```python
from build123d import *

# Parameters (mm, degrees)
SKETCH048_R     = 6.5
SKETCH048_R_2   = 3
PAD021_DEPTH    = 3.5
SKETCH049_R     = 5.5
SKETCH049_R_2   = 4
POCKET027_DEPTH = 0.5
SKETCH050_R     = 5.5
SKETCH050_R_2   = 4
POCKET028_DEPTH = 0.5


with BuildPart() as part:
    # Sketch048 → Pad021 (new body)
    with BuildSketch(Plane.XY):
        Circle(SKETCH048_R)
        Circle(SKETCH048_R_2, mode=Mode.SUBTRACT)
    extrude(amount=PAD021_DEPTH)

    # Sketch049 → Pocket027 (cut)
    with BuildSketch(Plane.XY.offset(3.5)):
        Circle(SKETCH049_R)
        Circle(SKETCH049_R_2, mode=Mode.SUBTRACT)
    extrude(amount=-POCKET027_DEPTH, mode=Mode.SUBTRACT)

    # Sketch050 → Pocket028 (cut)
    with BuildSketch(Plane.XY):
        Circle(SKETCH050_R)
        Circle(SKETCH050_R_2, mode=Mode.SUBTRACT)
    extrude(amount=POCKET028_DEPTH, mode=Mode.SUBTRACT)


solid = part.part
```
The listing builds one solid part. Answer for the finished solid, in the listing's coordinates (mm). A direction names the side the tool comes from. Give positions to 0.01 mm unless a question says otherwise; leave off trailing zeros. Order: outer loops, then holes, each group sorted by start corner. A loop starts at its lowest first (then second) coordinate and runs counter-clockwise, first axis right, second up.
1) Find section D-D on x = 4.25. Write down the section's boundary in (y, z), then the cut area to 3 significant figures.
Reported:
outline: (-4.92, 0) - (-3.49, 0) - (-3.49, 0.5) - (3.49, 0.5) - (3.49, 0) - (4.92, 0) - (4.92, 3.5) - (3.49, 3.5) - (3.49, 3) - (-3.49, 3) - (-3.49, 3.5) - (-4.92, 3.5) - close
area: 27.4 mm2
2) Consider line 1 along Y through (x, z) = (0, 0.35); line 2 along Z through (x, y) = (-5, 1.75); line 3 along X through (y, z) = (1.5, 3.1). Determine where each line is inside the solid, lowest interval first.
Reported:
line 1: y = -6.5 to -5.5, -4 to -3, 3 to 4, 5.5 to 6.5
line 2: z = 0.5 to 3
line 3: x = -6.32 to -5.29, -3.71 to -2.6, 2.6 to 3.71, 5.29 to 6.32
3) Given P1, Ø1, axis at y = -1, z = 1.5, coming from the +X side; P2, Ø1, axis at y = 1.5, z = 2.5, coming from the +X side; P3, Ø3.5, axis at x = 2, y = 2, coming from the -Z side, each flat-ended and moving along its own axis, determine where each tip first touches the part or whether it passes through.
Reported:
P1: stops at x = 6.48
P2: stops at x = 6.42
P3: stops at z = 0
4) Find section C-C on z = 3.2. Write down the section's boundary in (x, y).
Reported:
outline: circle Ø13 at (0, 0); circle Ø8 at (0, 0); hole circle Ø11 at (0, 0); hole circle Ø6 at (0, 0)
5) For faces 1 (the face through (-1.19, -5.37, 3.25)), 2 (the face through (-1.19, -5.37, 0.25)), 3 (the face through (1, 3, 0)), determine the directions among +Z, -Z, +X, -X, +Y, -Y from which every point of the face is accessible in a straight line to the end or side of a thin tool.
Reported:
face 1: +Z
face 2: -Z
face 3: -Z, +X, -X, +Y, -Y
6) Find section A-A on y = 0. Write down the section's boundary in (x, z), then the cut area to 3 significant figures.
Reported:
outline: (-6.5, 0) - (-5.5, 0) - (-5.5, 0.5) - (-4, 0.5) - (-4, 0) - (-3, 0) - (-3, 3.5) - (-4, 3.5) - (-4, 3) - (-5.5, 3) - (-5.5, 3.5) - (-6.5, 3.5) - close; (3, 0) - (4, 0) - (4, 0.5) - (5.5, 0.5) - (5.5, 0) - (6.5, 0) - (6.5, 3.5) - (5.5, 3.5) - (5.5, 3) - (4, 3) - (4, 3.5) - (3, 3.5) - close
area: 21.5 mm2
7) Determine the mould class of faces 4 (the face through (-4, -2, 3)), 5 (the face through (1, 3, 3.5)), 6 (the face through (-0.867, -3.905, 3.254)), 7 (the face through (-5.158, -3.955, 1.726)) for opening direction Y: pulls with the +Y half, pulls with the -Y half, needs draft (parallel to the pull), parting line crosses it, or undercut.
Reported:
face 4: undercut
face 5: needs draft
face 6: undercut
face 7: parting line crosses it
